```python
from build123d import *

# Parameters (mm, degrees)
F0_R     = 3.1
F0_R_2   = 3.6
F1_DEPTH = 30
F2_W     = 10
F2_H     = 4
F3_DEPTH = 40.001
F4_R     = 1
F5_R     = 3.6
F6_DEPTH = 25
F7_SIZE  = 2
F9_DEPTH = 46.6700476997


with BuildPart() as f1:
    # F0 (on Top) → F1 (new body)
    with BuildSketch(Plane.XY):
        with BuildLine():
            Line((16.4454364826, 19.4454364826), (-16.5545635174, 19.4454364826))
            ThreePointArc((-16.5545635174, 19.4454364826), (-19.3829906421, 18.2738636074), (-20.5545635174, 15.4454364826))
            Line((-20.5545635174, 15.4454364826), (-20.5545635174, 13.4454364826))
            ThreePointArc((-20.5545635174, 13.4454364826), (-19.3829906421, 10.6170093579), (-16.5545635174, 9.4454364826))
            Line((-16.5545635174, 9.4454364826), (-13.5545635174, 9.4454364826))
            ThreePointArc((-13.5545635174, 9.4454364826), (2.7088924499, 2.7088924499), (9.4454364826, -13.5545635174))
            Line((9.4454364826, -13.5545635174), (9.4454364826, -16.5545635174))
            ThreePointArc((9.4454364826, -16.5545635174), (10.6170093579, -19.3829906421), (13.4454364826, -20.5545635174))
            Line((13.4454364826, -20.5545635174), (15.4454364826, -20.5545635174))
            ThreePointArc((15.4454364826, -20.5545635174), (18.2738636074, -19.3829906421), (19.4454364826, -16.5545635174))
            Line((19.4454364826, -16.5545635174), (19.4454364826, 16.4454364826))
            ThreePointArc((19.4454364826, 16.4454364826), (18.5667568262, 18.5667568262), (16.4454364826, 19.4454364826))
        make_face()
        with Locations((14.4454364826, -13.5545635174)):
            Circle(F0_R, mode=Mode.SUBTRACT)
        with Locations((-13.5545635174, 14.4454364826)):
            Circle(F0_R, mode=Mode.SUBTRACT)
        with Locations((6.4454364826, 6.4454364826)):
            Circle(F0_R_2, mode=Mode.SUBTRACT)
    extrude(amount=F1_DEPTH)

    # F2 (on face) → F3 (cut, through all)
    with BuildSketch(Plane(origin=(0, 19.4454364826, 0), x_dir=(-1, 0, 0), z_dir=(0, 1, 0))):
        with Locations((13.5545635174, 28)):
            Rectangle(F2_W, F2_H)
        with Locations((13.5545635174, 2)):
            Rectangle(F2_W, F2_H)
    extrude(amount=-F3_DEPTH, mode=Mode.SUBTRACT)

    # F4
    f4_edges = [f1.edges().sort_by_distance(p)[0] for p in [
        (4.389795, 0.832931, 30),
        (-20.554564, 14.445436, 30),
        (-8.554564, 14.170409, 30),
    ]]
    fillet(f4_edges, radius=F4_R)

    # F5 (on face) → F6 (join)
    with BuildSketch(Plane(origin=(0, 0, 0), x_dir=(1, 0, 0), z_dir=(0, 0, -1))):
        with BuildLine():
            Line((-8.5545635174, 8.5545635174), (-8.5545635174, -19.4454364826))
            Line((-8.5545635174, -19.4454364826), (16.4454364826, -19.4454364826))
            ThreePointArc((16.4454364826, -19.4454364826), (18.5667568262, -18.5667568262), (19.4454364826, -16.4454364826))
            Line((19.4454364826, -16.4454364826), (19.4454364826, 8.5545635174))
            Line((19.4454364826, 8.5545635174), (-8.5545635174, 8.5545635174))
        make_face()
        with Locations((6.4454364826, -6.4454364826)):
            Circle(F5_R, mode=Mode.SUBTRACT)
    extrude(amount=F6_DEPTH)

    # F7
    f7_edges = [f1.edges().sort_by_distance(p)[0] for p in [
        (19.445436, -8.554564, -12.5),
        (-8.554564, 19.445436, -10.5),
    ]]
    chamfer(f7_edges, length=F7_SIZE)

    # F8 (on face) → F9 (cut, through all)
    with BuildSketch(Plane(origin=(13, -13, 0), x_dir=(0.7071067812, 0.7071067812, 0), z_dir=(0.7071067812, -0.7071067812, 0))):
        Polygon((16.1152236891, -4), (16.1152236891, 0), (-28.8847763109, 0), (-28.8847763109, -49), align=None)
    extrude(amount=-F9_DEPTH, mode=Mode.SUBTRACT)


solid = f1.part
```
Model file for the job. Use its own axes, mm. A direction names the side the tool comes from. Coordinates: 2 decimals unless noted, no trailing zeros. Loops run counter-clockwise (first coordinate to the right, second up) from the corner with the lowest first, then second, coordinate; pieces in that order, holes last. Notation, with made-up numbers: M -31.5,2.25 L -17.5,2.25 A18 ccw -17.5,37.25 Z; hole C -4.75,-8 d7. An arc over 180 degrees is marked long. Use CSV: the item, a comma, the result in double quotes. Start each with the question number.
1. Two-plate mould, pull along X, no slides. Class faces 1 (the flat face through (19.445, 4, 2)), 2 (the flat face through (13, -8.555, -22)), 3 (the cylindrical face through (8.107, 9.639, -17.957)): pulls with the +X half, pulls with the -X half, needs draft (parallel to the pull), parting line crosses it, or undercut.
2. Probe probe 1 along Z at (x, y) = (-3, 13.5); probe 2 along Z at (x, y) = (7, 1.5); probe 3 along X at (y, z) = (15, 6). List the from-to ranges inside material, lowest first. Write a range as [from, to].
3. Band-saw the part on D-D, the plane y = 5.5. Give the number of separate pieces and of enclosed holes in the cut face, then the cut area to 3 significant figures.
4. Band-saw the part on C-C, the plane z = -15. List the corners of the cut face in (x, y).
5. Band-saw the part on A-A, the plane x = -15. List the corners of the cut face in (y, z), then the cut area to 3 significant figures.
6. Flat gauge pins, fed straight in: pin 1 (9.5 mm diameter, centred on x = 6.45, y = 6.45, fed in from -Z); pin 2 (11.5 mm diameter, centred on x = -14.5, y = 15.5, fed in from -Z); pin 3 (1.5 mm diameter, centred on y = 2.5, z = -14.5, fed in from -X); pin 4 (12.5 mm diameter, centred on x = 11, z = -18, fed in from -Y). Where does each tip first touch, or does it go through?
7. Band-saw the part on B-B, the plane z = 18.5. List the corners of the cut face in (x, y), then the cut area to 3 significant figures.
8. Tool access for faces 4 (the flat face through (-18.555, 15, 28)), 5 (the flat face through (-18.555, 15, 2)), 6 (the flat face through (1.2, 6.6, -14.6)): list every direction of +Z, -Z, +X, -X, +Y, -Y with a clear straight run to the whole face (end or side of a thin tool).
Entries:
1,face 1,"pulls with the +X half"
1,face 2,"needs draft"
1,face 3,"undercut"
2,probe 1,"z = [-25, -12.69], [0, 30]"
2,probe 2,"z = [-25, -14.1], [0, 30]"
2,probe 3,"x = [-20.55, -16.6], [-10.5, 19.45]"
3,separate pieces,"3"
3,enclosed holes,"0"
3,area,"662 mm2"
4,outline,"M -8.55,15.79 L 15.79,-8.55 L 17.45,-8.55 L 19.45,-6.55 L 19.45,16.45 A3 ccw 16.45,19.45 L -6.55,19.45 L -8.55,17.45 Z; hole C 6.45,6.45 d7.2"
5,outline,"M 9.45,4 L 11.7,4 L 11.7,26 L 9.45,26 Z; M 17.19,4 L 19.45,4 L 19.45,26 L 17.19,26 Z"
5,area,"99.3 mm2"
6,pin 1,"stops at z = -25"
6,pin 2,"stops at z = 0"
6,pin 3,"stops at x = 4.14"
6,pin 4,"stops at y = -8.55"
7,outline,"M -20.55,13.45 A4 ccw -16.55,9.45 L -13.55,9.45 A23 cw 9.45,-13.55 L 9.45,-16.55 A4 ccw 13.45,-20.55 L 15.45,-20.55 A4 ccw 19.45,-16.55 L 19.45,16.45 A3 ccw 16.45,19.45 L -16.55,19.45 A4 ccw -20.55,15.45 Z; hole C -13.55,14.45 d6.2; hole C 6.45,6.45 d7.2; hole C 14.45,-13.55 d6.2"
7,area,"697 mm2"
8,face 4,"+Z, +Y, -Y"
8,face 5,"-Z, +Y, -Y"
8,face 6,"-X, -Y"
